```python
from build123d import *

# Parameters (mm, degrees)
CORTAR_EXTRUIR1_DEPTH = 18.374694242


with BuildPart() as part:
    # Croquis3 → Revolución1 (revolve)
    with BuildSketch(Plane.XY):
        Polygon((3.2, 0), (6.2, 0), (6.2, 15), (2.75, 15), (2.75, 27), (0, 27), (0, 13), (3.2, 13), align=None)
    revolve(axis=Axis((0, -169.632312065, 0), (0, 1, 0)))

    # Croquis4 → Cortar-Extruir1 (cut, through all)
    with BuildSketch(Plane(origin=(0, 15, 0), x_dir=(1, 0, 0), z_dir=(0, 1, 0))):
        with BuildLine():
            Line((1.85, 2.034698995), (1.85, -2.034698995))
            ThreePointArc((1.85, -2.034698995), (2.75, 0), (1.85, 2.034698995))
        make_face()
        with BuildLine():
            Line((-1.85, 2.034698995), (-1.85, -2.034698995))
            ThreePointArc((-1.85, -2.034698995), (-2.75, 0), (-1.85, 2.034698995))
        make_face()
    extrude(amount=CORTAR_EXTRUIR1_DEPTH, mode=Mode.SUBTRACT)


solid = part.part
```
For this review, take the finished solid that the model builds, in its own axes (mm). A direction names the side the tool comes from. Coordinates: 2 decimals unless noted, no trailing zeros. Loops run counter-clockwise (first coordinate to the right, second up) from the corner with the lowest first, then second, coordinate; pieces in that order, holes last. Notation, with made-up numbers: (61.25, 52) -> (86.25, 52) arc R15 cw to (86.25, 73) -> close; hole circle Ø10 at (9, -14). An arc over 180 degrees is marked (long way). Return JSON: item names as keys, results as strings. Group by question number.
(1) Consider section A-A, the plane z = 0. Give the boundary of the cut face in (x, y).
(2) Consider section C-C, the plane y = 12.5. Give the boundary of the cut face in (x, z), plus the area to 3 significant figures.
(3) For pin 1 Ø1.9 at (x, z) = (0.5, 1) entering from -Y; pin 2 Ø6 at (y, z) = (19, -1.5) entering from +X; pin 3 Ø2 at (x, y) = (-0.5, 17.5) entering from -Z; pin 4 Ø2 at (x, y) = (-4.5, 24) entering from +Z, all flat-tipped, find the tip position at first contact; note any pin that passes through.
(4) Tool access review of faces 1 (the cylindrical face through (0.03, 21.08, -2.75)), 2 (the flat face through (-1.85, 21, 0)), 3 (the cylindrical face through (-2.539, 6.409, 1.947)): name each direction out of +Z, -Z, +X, -X, +Y, -Y from which nothing blocks a thin tool from reaching the whole face with its end or side.
(5) Mouldability with a two-part tool opening along X and no side actions: class faces 4 (the flat face through (1.85, 21, 0)), 5 (the flat face through (0, 27, 0)), 6 (the flat face through (0, 13, 0)) as pulls with the +X half, pulls with the -X half, needs draft (parallel to the pull), parting line crosses it, or undercut.
(6) To check wall thickness, follow L1, parallel to X at y = 9, z = 0; L2, parallel to Y at x = -4, z = 2.25. State the ranges of each line that lie inside material, in increasing order.
(7) Consider section D-D, the plane y = 21.5. Give the boundary of the cut face in (x, z).
(8) Consider section B-B, the plane x = 0. Give the boundary of the cut face in (y, z), plus the area to 3 significant figures.
Results below:
{
 "1": {"outline": "(-6.2, 0) -> (-3.2, 0) -> (-3.2, 13) -> (3.2, 13) -> (3.2, 0) -> (6.2, 0) -> (6.2, 15) -> (1.85, 15) -> (1.85, 27) -> (-1.85, 27) -> (-1.85, 15) -> (-6.2, 15) -> close"},
 "2": {"outline": "circle Ø12.4 at (0, 0); hole circle Ø6.4 at (0, 0)", "area": "88.6 mm2"},
 "3": {"pin 1": "stops at y = 13", "pin 2": "stops at x = 1.85", "pin 3": "stops at z = -2.75", "pin 4": "passes through"},
 "4": {"face 1": "-Z, +Y", "face 2": "+Z, -Z, -X, +Y", "face 3": "-Y"},
 "5": {"face 4": "pulls with the +X half", "face 5": "needs draft", "face 6": "undercut"},
 "6": {"L1": "x = -6.2 to -3.2, 3.2 to 6.2", "L2": "y = 0 to 15"},
 "7": {"outline": "(-1.85, -2.03) arc R2.75 ccw to (1.85, -2.03) -> (1.85, 2.03) arc R2.75 ccw to (-1.85, 2.03) -> close"},
 "8": {"outline": "(0, -6.2) -> (15, -6.2) -> (15, -2.75) -> (27, -2.75) -> (27, 2.75) -> (15, 2.75) -> (15, 6.2) -> (0, 6.2) -> (0, 3.2) -> (13, 3.2) -> (13, -3.2) -> (0, -3.2) -> close", "area": "169 mm2"}
}
